```python
from build123d import *

# Parameters (mm, degrees)
SKETCH1_W           = 70
SKETCH1_H           = 70
SKETCH1_R           = 1.35
BOSS_EXTRUDE1_DEPTH = 5
FILLET1_R           = 1.5
SKETCH2_W           = 24.359680225
SKETCH2_H           = 19.606300568
BOSS_EXTRUDE2_DEPTH = 9


with BuildPart() as part:
    # Sketch1 → Boss-Extrude1 (new body)
    with BuildSketch(Plane.XY):
        Rectangle(SKETCH1_W, SKETCH1_H)
        with Locations((-32.84, 32.82)):
            Circle(SKETCH1_R, mode=Mode.SUBTRACT)
        with Locations((-32.84, -32.84)):
            Circle(SKETCH1_R, mode=Mode.SUBTRACT)
        with Locations((32.82, -32.84)):
            Circle(SKETCH1_R, mode=Mode.SUBTRACT)
        with Locations((32.82, 32.82)):
            Circle(SKETCH1_R, mode=Mode.SUBTRACT)
    extrude(amount=BOSS_EXTRUDE1_DEPTH)

    # Fillet1
    fillet1_edges = [part.edges().sort_by_distance(p)[0] for p in [
        (35, -35, 2.5),
        (-35, -35, 2.5),
        (-35, 35, 2.5),
        (35, 35, 2.5),
    ]]
    fillet(fillet1_edges, radius=FILLET1_R)

    # Sketch2 → Boss-Extrude2 (add)
    with BuildSketch(Plane(origin=(0, 0, 0), x_dir=(-1, 0, 0), z_dir=(0, 0, -1))):
        with Locations((1.199225338, -25.196849716)):
            Rectangle(SKETCH2_W, SKETCH2_H)
    extrude(amount=BOSS_EXTRUDE2_DEPTH)


solid = part.part
```
Geometry: final body of the model. Coordinates: model frame, mm. A direction names the side the tool comes from. Coordinates: 2 decimals unless noted, no trailing zeros. Order: outer loops, then holes, each group sorted by start corner. A loop starts at its lowest first (then second) coordinate and runs counter-clockwise, first axis right, second up. Notation, with made-up numbers: (77.25, -16.5) - (94.25, -16.5) arc R14 cw to (94.25, -8.5) - close; hole circle Ø10 at (18, -27.5). An arc over 180 degrees is marked (long way). Write each question's results on one line, items separated by ' | '.
(1) Section query A-A, the plane z = -6.5. Return the cut outline in (x, y), plus the area to 3 significant figures.
Values found:
outline: (-13.38, -35) - (10.98, -35) - (10.98, -15.39) - (-13.38, -15.39) - close | area: 478 mm²
(2) Set-up query: faces 1 (the face through (-13.379, -25, -4)), 2 (the face through (-34.19, -32.78, 2.46)), 3 (the face through (-1, -15.394, -4)), 4 (the face through (10.981, -25, -4)). Return all of +Z, -Z, +X, -X, +Y, -Y with unobstructed straight access to the full face (end or side cutting, diameter ignored); none if empty.
Values found:
face 1: -Z, -X, +Y, -Y | face 2: +Z, -Z | face 3: -Z, +X, -X, +Y | face 4: -Z, +X, +Y, -Y
(3) Line query: line 1 (Y direction, x = 32.82, z = 2.5); line 2 (Z direction, x = 20, y = -6); line 3 (X direction, y = -22, z = -1). Output: solid intervals per line, ascending. Write a range as [from, to].
Values found:
line 1: y = [-35, -34.19], [-31.49, 31.47], [34.17, 35] | line 2: z = [0, 5] | line 3: x = [-13.38, 10.98]
(4) Section query B-B, the plane x = -16. Return the cut outline in (y, z).
Values found:
outline: (-35, 0) - (35, 0) - (35, 5) - (-35, 5) - close
(5) Mould query, pull axis Y, two halves, no side actions, for faces 5 (the face through (34.067, -33.357, 2.465)), 6 (the face through (33.546, 33.958, 2.465)), 7 (the face through (-34.57, -34.55, 2.54)), 8 (the face through (35, 0, 2)). Classes: +Y half, -Y half, draft (parallel to the pull), parting line (faces both ways), or undercut.
Values found:
face 5: undercut | face 6: undercut | face 7: -Y half | face 8: draft
(6) First-contact query: pin 1 Ø3 at (x, y) = (-32.84, -32.84) entering from -Z; pin 2 Ø2.5 at (y, z) = (-29, -4) entering from -X; pin 3 Ø2 at (x, y) = (32.82, -32.84) entering from -Z. Flat tips, straight axial feed; report the tip coordinate or a pass-through.
Values found:
pin 1: stops at z = 0 | pin 2: stops at x = -13.38 | pin 3: passes through
